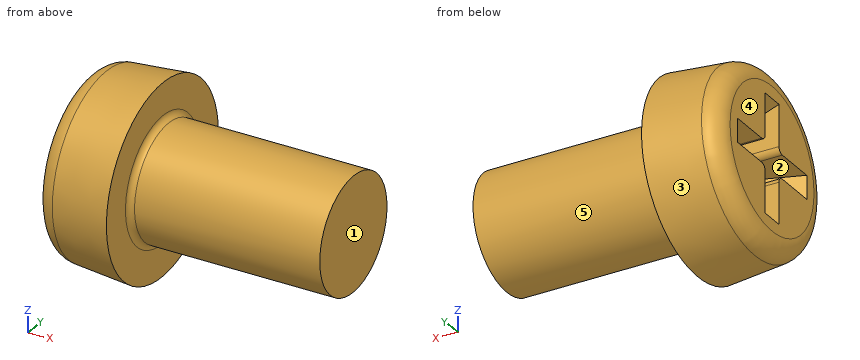
```python
from build123d import *

# Parameters (mm, degrees)
CROSSRECESS_DEPTH = 3.9
FILLET5_R         = 0.3
HEADFILLET_R      = 1
DRAFT1_ANGLE      = 20


with BuildPart() as part:
    # Sketch1 → Base (revolve)
    with BuildSketch(Plane.XY):
        with BuildLine():
            Line((13.9, 3), (5.9, 3))
            Line((5.9, 3), (4.2, 3))
            ThreePointArc((4.2, 3), (3.987867966, 3.087867966), (3.9, 3.3))
            Line((3.9, 3.3), (3.9, 5))
            Line((3.9, 5), (0, 4.658794212))
            Line((0, 4.658794212), (0, 0))
            Line((0, 0), (13.9, 0))
            Line((13.9, 0), (13.9, 3))
        make_face()
    revolve(axis=Axis((4.515812911, 0, 0), (-1, 0, 0)))

    # Sketch6 → CrossRecess (cut)
    with BuildSketch(Plane(origin=(0, 0, 0), x_dir=(0, 0, -1), z_dir=(1, 0, 0))):
        Polygon((0.62, 0.62), (0.62, 3.1), (-0.62, 3.1), (-0.62, 0.62), (-3.1, 0.62), (-3.1, -0.62), (-0.62, -0.62), (-0.62, -3.1), (0.62, -3.1), (0.62, -0.62), (3.1, -0.62), (3.1, 0.62), align=None)
    extrude(amount=CROSSRECESS_DEPTH, mode=Mode.SUBTRACT)

    # Fillet5
    fillet5_edges = [part.edges().sort_by_distance(p)[0] for p in [
        (1.95, 0.62, 0.62),
        (1.95, -0.62, 0.62),
        (1.95, -0.62, -0.62),
        (1.95, 0.62, -0.62),
    ]]
    fillet(fillet5_edges, radius=FILLET5_R)

    # HeadFillet
    headfillet_edges = [part.edges().sort_by_distance(p)[0] for p in [
        (0, -4.658794212, 0),
    ]]
    fillet(headfillet_edges, radius=HEADFILLET_R)

    # Draft1
    draft1_faces = [part.faces().sort_by_distance(p)[0] for p in [
        (1.95, 0, 3.1),
        (1.95, -3.1, 0),
        (1.95, 0, -3.1),
        (1.95, 3.1, 0),
    ]]
    draft(draft1_faces, Plane(origin=(0, 0, 0), x_dir=(0, 0, -1), z_dir=(-1, 0, 0)), DRAFT1_ANGLE)


solid = part.part
```
Verification items for the finished model (mm, model axes). Face numbers are marked on the shaded views. A direction names the side the tool comes from. Round coordinates to 2 decimals unless told otherwise and drop trailing zeros. Loops run counter-clockwise (first coordinate to the right, second up) from the corner with the lowest first, then second, coordinate; pieces in that order, holes last. Notation, with made-up numbers: (-26.75, 12.5) -> (21.25, 12.5) arc R9 cw to (21.25, 17.5) -> close; hole circle Ø10 at (-29, 58). An arc over 180 degrees is marked (long way). Answer as a JSON object with one key per item and string values.
Q1. Access from +Z, -Z, +X, -X, +Y, -Y to the whole of each face (thin tool, end or side, straight path). Record for the marked faces 4 and 5.
Data:
{"face 4": "+Z, -Z, -X, +Y, -Y", "face 5": "+X"}
Q2. Section check D-D (x = 1.5). Record the boundary of the cut face in (y, z), then the cut area to 3 significant figures.
Data:
{"outline": "circle Ø9.58 at (0, 0); hole (-2.55, -0.62) -> (-0.92, -0.62) arc R0.3 cw to (-0.62, -0.92) -> (-0.62, -2.55) -> (0.62, -2.55) -> (0.62, -0.92) arc R0.3 cw to (0.92, -0.62) -> (2.55, -0.62) -> (2.55, 0.62) -> (0.92, 0.62) arc R0.3 cw to (0.62, 0.92) -> (0.62, 2.55) -> (-0.62, 2.55) -> (-0.62, 0.92) arc R0.3 cw to (-0.92, 0.62) -> (-2.55, 0.62) -> close", "area": "60.9 mm2"}
Q3. Section check C-C (x = 10). Record the boundary of the cut face in (y, z), then the cut area to 3 significant figures.
Data:
{"outline": "circle Ø6 at (0, 0)", "area": "28.3 mm2"}
Q4. Go/stop test with flat-tipped pins: P1, Ø0.7, axis at x = 3, z = 2, coming from the +Y side; P2, Ø0.7, axis at x = 1.5, z = 2.5, coming from the -Y side; P3, Ø2.5, axis at x = 2.5, z = -1.5, coming from the -Y side. Record where each tip stops, or that it passes through.
Data:
{"P1": "stops at y = 4.64", "P2": "stops at y = -4.28", "P3": "stops at y = -4.92"}
Q5. Scan lines: line 1 (X direction, y = -3.5, z = -0.25); line 2 (X direction, y = -0.5, z = 0.75); line 3 (Z direction, x = 3, y = -0.75). Record each from-to range of solid material in increasing order. Write a range as from..to.
Data:
{"line 1": "x = 0..3.9", "line 2": "x = 3.9..13.9", "line 3": "z = -4.86..-0.67, 0.67..4.86"}
Q6. Section check A-A (y = 0). Record the boundary of the cut face in (x, z), then the cut area to 3 significant figures.
Data:
{"outline": "(0, -3.74) arc R1 ccw to (0.91, -4.74) -> (3.9, -5) -> (3.9, -3.3) arc R0.3 cw to (4.2, -3) -> (13.9, -3) -> (13.9, 3) -> (4.2, 3) arc R0.3 cw to (3.9, 3.3) -> (3.9, 5) -> (0.91, 4.74) arc R1 ccw to (0, 3.74) -> (0, 3.1) -> (3.9, 1.68) -> (3.9, -1.68) -> (0, -3.1) -> close", "area": "78.7 mm2"}
Q7. Draft check along Y on the marked faces 1, 2 and 3. Enter one of: pulls with the +Y half, pulls with the -Y half, needs draft (parallel to the pull), parting line crosses it, or undercut.
Data:
{"face 1": "needs draft", "face 2": "undercut", "face 3": "parting line crosses it"}
